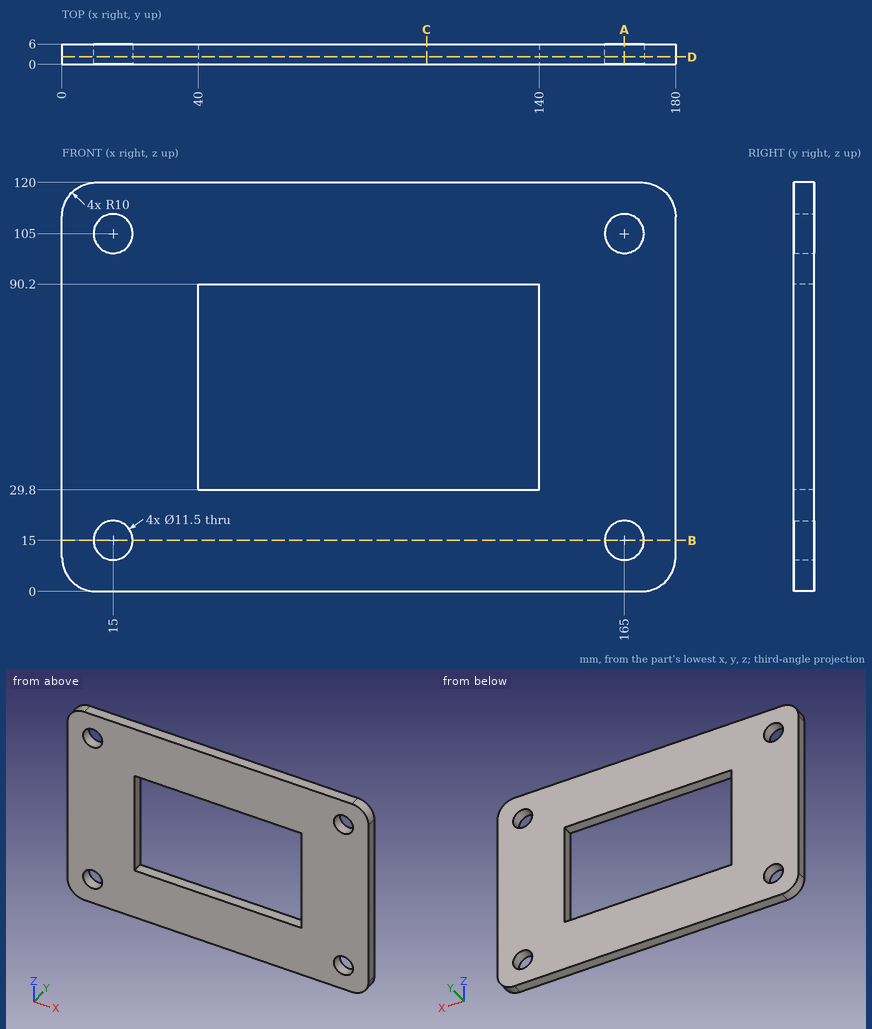
Print and shaded views of the part. All mm, measured from the part's lowest x, y and z. Coordinates: 2 decimals unless noted, no trailing zeros. Order: outer loops, then holes, each group sorted by start corner. A loop starts at its lowest first (then second) coordinate and runs counter-clockwise, first axis right, second up. Notation, with made-up numbers: (-38, -32) -> (11, -32) arc R26 ccw to (11, -4) -> close; hole circle Ø8 at (66, 15). An arc over 180 degrees is marked (long way). Use one line per item in the form item = value. Start each with the question number.
1) Drop a flat-ended pin along its axis: pin 1 (10.5 mm diameter, centred on x = 165, z = 15, fed in from -Y). Give the stop position or say it passes through.
2) Drill centre lines: L1, parallel to Z at x = 165, y = 1.2; L2, parallel to Z at x = 60, y = 3.2; L3, parallel to X at y = 0.95, z = 45. Where is each one in solid material? Low to high. Write a range as [from, to].
3) Band-saw the part on A-A on x = 165. Give the cut face in (y, z), then the cut area to 3 significant figures.
4) Band-saw the part on B-B on z = 15. Give the cut face in (x, y), then the cut area to 3 significant figures.
5) Band-saw the part on D-D on y = 2.2. Give the cut face in (x, z), then the cut area to 3 significant figures.
6) Band-saw the part on C-C on x = 107. Give the cut face in (y, z), then the cut area to 3 significant figures.
Entries:
q1.pin_1 = through
q2.L1 = [0, 9.25], [20.75, 99.25], [110.75, 120]
q2.L2 = [0, 29.8], [90.2, 120]
q2.L3 = [0, 40], [140, 180]
q3.outline = (0, 0) -> (6, 0) -> (6, 9.25) -> (0, 9.25) -> close; (0, 20.75) -> (6, 20.75) -> (6, 99.25) -> (0, 99.25) -> close; (0, 110.75) -> (6, 110.75) -> (6, 120) -> (0, 120) -> close
q3.area = 582 mm2
q4.outline = (0, 0) -> (9.25, 0) -> (9.25, 6) -> (0, 6) -> close; (20.75, 0) -> (159.25, 0) -> (159.25, 6) -> (20.75, 6) -> close; (170.75, 0) -> (180, 0) -> (180, 6) -> (170.75, 6) -> close
q4.area = 942 mm2
q5.outline = (0, 10) arc R10 ccw to (10, 0) -> (170, 0) arc R10 ccw to (180, 10) -> (180, 110) arc R10 ccw to (170, 120) -> (10, 120) arc R10 ccw to (0, 110) -> close; hole circle Ø11.5 at (15, 15); hole circle Ø11.5 at (15, 105); hole (40, 29.8) -> (140, 29.8) -> (140, 90.2) -> (40, 90.2) -> close; hole circle Ø11.5 at (165, 15); hole circle Ø11.5 at (165, 105)
q5.area = 15,100 mm2
q6.outline = (0, 0) -> (6, 0) -> (6, 29.8) -> (0, 29.8) -> close; (0, 90.2) -> (6, 90.2) -> (6, 120) -> (0, 120) -> close
q6.area = 358 mm2
